```python
from build123d import *

# Parameters (mm, degrees)
BOSS_EXTRUDE1_DEPTH        = 9.525
F_10_32_TAPPED_HOLE2_D     = 4.0386
F_10_32_TAPPED_HOLE2_DEPTH = 14.5796
F_6_0_204_DIAMETER_HOLE1_D = 5.1816


with BuildPart() as part:
    # Sketch1 → Boss-Extrude1 (new body)
    with BuildSketch(Plane.XY):
        with BuildLine():
            Line((-63.3222, 0), (-63.3222, -66.4972))
            Line((-63.3222, -66.4972), (63.3222, -66.4972))
            Line((63.3222, -66.4972), (63.3222, 0))
            ThreePointArc((63.3222, 0), (60.350483171, 19.170816203), (51.714258587, 36.542255974))
            ThreePointArc((51.714258587, 36.542255974), (51.142998099, 38.702969527), (52.124965643, 40.710645135))
            Line((52.124965643, 40.710645135), (57.191705625, 45.518801846))
            Line((57.191705625, 45.518801846), (52.820654069, 50.124929102))
            Line((52.820654069, 50.124929102), (41.32617374, 39.217074557))
            ThreePointArc((41.32617374, 39.217074557), (-40.285428959, -40.285428959), (39.217074557, 41.32617374))
            Line((39.217074557, 41.32617374), (50.124929102, 52.820654069))
            Line((50.124929102, 52.820654069), (45.518801846, 57.191705625))
            Line((45.518801846, 57.191705625), (40.710645135, 52.124965643))
            ThreePointArc((40.710645135, 52.124965643), (38.702969527, 51.142998099), (36.542255974, 51.714258587))
            ThreePointArc((36.542255974, 51.714258587), (-29.11842176, 56.230050036), (-63.3222, 0))
        make_face()
    extrude(amount=BOSS_EXTRUDE1_DEPTH)

    # #10-32 Tapped Hole2
    with Locations(Plane(origin=(0, -66.4972, 0), x_dir=(-1, 0, 0), z_dir=(0, -1, 0))):
        with Locations((-41.275, -4.7625), (41.275, -4.7625)):
            Hole(F_10_32_TAPPED_HOLE2_D / 2, depth=F_10_32_TAPPED_HOLE2_DEPTH)

    # #6 (0.204) Diameter Hole1 (through all)
    with Locations(Plane(origin=(54.658335634, 43.114723491, 4.7625), x_dir=(-0.725374371012, -0.688354575694, 0), z_dir=(0.688354575694, -0.725374371012, 0))):
        with Locations((0, 0)):
            Hole(F_6_0_204_DIAMETER_HOLE1_D / 2)


solid = part.part
```
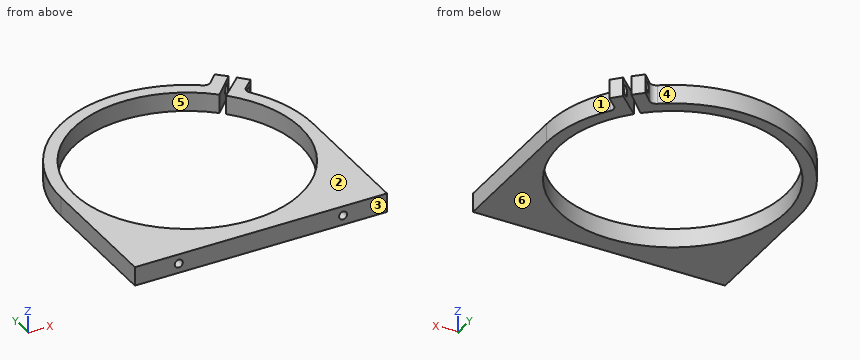
Input: part model. Units: mm. Frame: model coordinates. Face numbers are marked on the shaded views. A direction names the side the tool comes from. Give positions to 0.01 mm unless a question says otherwise; leave off trailing zeros. Order: outer loops, then holes, each group sorted by start corner. A loop starts at its lowest first (then second) coordinate and runs counter-clockwise, first axis right, second up. Notation, with made-up numbers: (16.25, 81.25) - (65.25, 81.25) arc R24 cw to (65.25, 93.25) - close; hole circle Ø4 at (-25.75, 34). An arc over 180 degrees is marked (long way). Put each result on its own line as item: value.
Item 1: Section query A-A, the plane x = 0. Return loops of the section in (y, z) (3 decimals).
Found:
outline: (-66.497, 0) - (-56.972, 0) - (-56.972, 9.525) - (-66.497, 9.525) - close; (56.972, 0) - (63.322, 0) - (63.322, 9.525) - (56.972, 9.525) - close
Item 2: Draft query along Y for the marked faces 3, 4, 5 and 6. Return one class per face: +Y half, -Y half, draft (parallel to the pull), parting line (faces both ways), or undercut.
Found:
face 3: -Y half
face 4: +Y half
face 5: undercut
face 6: draft
Item 3: Contact query for flat-ended pins moving along their axis: pin 1 (2 mm diameter, centred on x = -8, z = 7.5, fed in from +Y); pin 2 (3.5 mm diameter, centred on x = -41.28, z = 4.76, fed in from -Y); pin 3 (3 mm diameter, centred on x = -31.5, z = 7.5, fed in from +Y). Output: stop coordinate, or through.
Found:
pin 1: stops at y = 62.93
pin 2: stops at y = -51.92
pin 3: stops at y = 55.76
Item 4: Section query B-B, the plane y = 32.5. Return loops of the section in (x, z) (3 decimals).
Found:
outline: (-54.346, 0) - (-46.793, 0) - (-46.793, 9.525) - (-54.346, 9.525) - close; (46.793, 0) - (54.346, 0) - (54.346, 9.525) - (46.793, 9.525) - close
Item 5: Ray query, L1, parallel to Y at x = 0, z = 4.5; L2, parallel to X at y = 44.5, z = 3; L3, parallel to X at y = 1, z = 9.25. Return the intervals inside material, ascending. Write a range as from..to.
Found:
L1: y = -66.5..-56.97, 56.97..63.32
L2: x = -45.05..-35.58, 35.58..42.23, 46.89..50.73, 55.96..56.12
L3: x = -63.31..-56.96, 56.96..63.31
Item 6: Access query for the marked faces 1 and 2. Directions: +Z, -Z, +X, -X, +Y, -Y. A direction counts if a zero-diameter tool reaches every point of the face in a straight line with its end or side. Return the directions, or none.
Found:
face 1: +Z, -Z, +X
face 2: +Z, +X, -X, +Y, -Y
